The model under review builds one solid part; all positions refer to its coordinate system, in mm. Give positions to 0.01 mm unless a question says otherwise; leave off trailing zeros. Loops run counter-clockwise (first coordinate to the right, second up) from the corner with the lowest first, then second, coordinate; pieces in that order, holes last. Notation, with made-up numbers: (-7.75, 76.5) - (-2.75, 76.5) arc R27 cw to (-2.75, 105.5) - close; hole circle Ø5 at (40.25, 1.25). An arc over 180 degrees is marked (long way). Return JSON: item names as keys, results as strings. Group by question number.
Autodesk Inventor part; units mm, degrees
ref_plane "YZ Plane" through (0, 0, 0) normal (1, 0, 0) x (0, 1, 0)
ref_plane "XZ Plane" through (0, 0, 0) normal (0, 1, 0) x (-1, 0, 0)
ref_plane "XY Plane" through (0, 0, 0) normal (0, 0, 1) x (1, 0, 0)
sketch "Sketch1" plane through (0, 0, 0) normal (0, 0, 1) x (1, 0, 0)
  line L0 (-7.5692, 0) -> (42.4308, 0)
  line L1 (42.4308, 0) -> (42.4308, 10)
  line L2 (-7.5692, 0) -> (-7.5692, 10)
  arc A0 (-7.5692, 10) -> (42.4308, 10) centre (17.4308, 132.4745) ccw
  point P0 (0, 0)
  dimension "d1" = 50
  dimension "d2" = 10
  dimension "d3" = 10
  dimension "d4" = 250
extrude "Extrusion1" add sketch "Sketch1" along normal blind 20
sketch "Sketch2" plane through (-7.5692, 0, 0) normal (0, -1, 0) x (1, 0, 0)
  line L0 (0, 0) -> (50, 0)
  point P0 (7.5692, 0)
  point P1 (25, 10)
  dimension "d7" = 10
hole "Hole1" at (17.4308, 0, 10) direction (0, 1, 0) diameter 6.756 end through all
properties part number "podkladka" material "ABS Plastic"
1) To check wall thickness, follow line 1 (X direction, y = 6.5, z = 10); line 2 (X direction, y = 4.5, z = 8.75); line 3 (Y direction, x = 21, z = 4.5). State the ranges of each line that lie inside material, in increasing order.
2) For pin 1 Ø5 at (x, z) = (22.5, 16) entering from +Y; pin 2 Ø2 at (x, z) = (30, 10) entering from +Y, all flat-tipped, find the tip position at first contact; note any pin that passes through.
3) Draft analysis for pull direction Z (two halves, no side actions). For faces 1 (the face through (14.08, 3.81, 10.44)), 2 (the face through (42.431, 5, 10)), 3 (the face through (17, 4, 0)), state which applies: +Z half, -Z half, draft (parallel to the pull), parting line (faces both ways), or undercut.
4) We need section D-D, the plane z = 1.75. Write out the cut boundary in (x, y).
5) We need section B-B, the plane y = 9.5. Write out the cut boundary in (x, z), plus the area to 3 significant figures.
6) We need section A-A, the plane z = 10. Write out the cut boundary in (x, y), plus the area to 3 significant figures.
7) We need section C-C, the plane y = 1.75. Write out the cut boundary in (x, z).
Findings:
{
 "1": {"line 1": "x = -7.57 to 14.05, 20.81 to 42.43", "line 2": "x = -7.57 to 14.29, 20.57 to 42.43", "line 3": "y = 0 to 7.53"},
 "2": {"pin 1": "stops at y = 7.7", "pin 2": "stops at y = 8.21"},
 "3": {"face 1": "undercut", "face 2": "draft", "face 3": "-Z half"},
 "4": {"outline": "(-7.57, 0) - (42.43, 0) - (42.43, 10) arc R125 cw to (-7.57, 10) - close"},
 "5": {"outline": "(-7.57, 0) - (-4.98, 0) - (-4.98, 20) - (-7.57, 20) - close; (39.84, 0) - (42.43, 0) - (42.43, 20) - (39.84, 20) - close", "area": "104 mm^2"},
 "6": {"outline": "(-7.57, 0) - (14.05, 0) - (14.05, 7.52) arc R125 cw to (-7.57, 10) - close; (20.81, 0) - (42.43, 0) - (42.43, 10) arc R125 cw to (20.81, 7.52) - close", "area": "365 mm^2"},
 "7": {"outline": "(-7.57, 0) - (42.43, 0) - (42.43, 20) - (-7.57, 20) - close; hole circle Ø6.76 at (17.43, 10)"}
}
